Here's how the part is built. I have some questions about the finished solid (model axes, mm). Face numbers are marked on the shaded views. A direction names the side the tool comes from. Round coordinates to 2 decimals unless told otherwise and drop trailing zeros. Loops run counter-clockwise (first coordinate to the right, second up) from the corner with the lowest first, then second, coordinate; pieces in that order, holes last. Notation, with made-up numbers: M 20,47.5 L 44,47.5 A6 cw 44,52.5 Z; hole C 42.25,28.5 d4. An arc over 180 degrees is marked long. Write item = value, one per line. Start each with the question number.
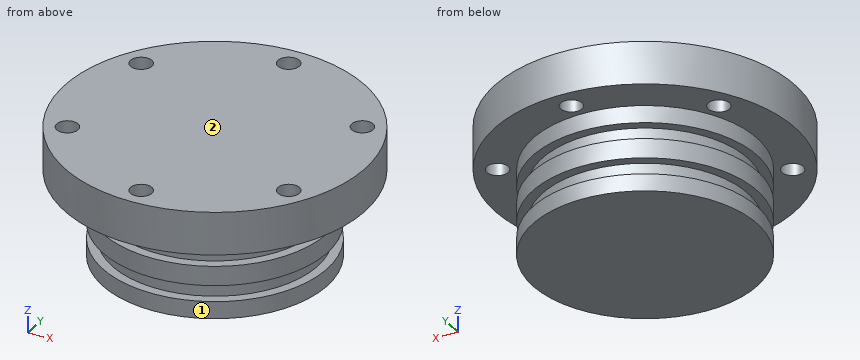
from build123d import *

# Parameters (mm, degrees)
F3_R     = 3.175
F4_DEPTH = 25.4


with BuildPart() as f2:
    # F0 (on Front) → F2 (revolve)
    with BuildSketch(Plane.XZ):
        Polygon((44.45, 38.1), (0, 38.1), (0, 0), (33.2105, 0), (33.2105, 5.08), (30.3911, 5.08), (30.3911, 9.8298), (33.2105, 9.8298), (33.2105, 15.5702), (30.3911, 15.5702), (30.3911, 20.32), (33.2105, 20.32), (33.2105, 25.4), (44.45, 25.4), align=None)
    revolve(axis=Axis((0, 0, 36.677974), (0, 0, -1)))

    # F3 (on face) → F4 (cut)
    with BuildSketch(Plane.XY.offset(38.1)):
        with Locations((0, -38.1)):
            Circle(F3_R)
        with Locations((32.995568, -19.05)):
            Circle(F3_R)
        with Locations((32.995568, 19.05)):
            Circle(F3_R)
        with Locations((0, 38.1)):
            Circle(F3_R)
        with Locations((-32.995568, 19.05)):
            Circle(F3_R)
        with Locations((-32.995568, -19.05)):
            Circle(F3_R)
    extrude(amount=-F4_DEPTH, mode=Mode.SUBTRACT)


solid = f2.part
Item 1: I want a section at C-C, the plane y = 0. List the corners of the cut face in (x, z) for me.
Item 2: I want a section at D-D, the plane x = 32. List the corners of the cut face in (y, z) for me.
Item 3: Will these pins go through, and if not, where does the flat tip stop? pin 1 Ø12 at (y, z) = (2, 13) entering from -X; pin 2 Ø2 at (y, z) = (16, 12) entering from +X; pin 3 Ø4 at (y, z) = (-20.5, 30.5) entering from +X.
Item 4: Please list where these lines run through material, in increasing order: line 1 (Z direction, x = 15.5, y = -28); line 2 (Y direction, x = 0, z = 28.75) (3 decimals); line 3 (X direction, y = -19, z = 30). Write a range as [from, to].
Item 5: I want a section at A-A, the plane x = 0. State how many separate pieces and enclosed holes the cut face has, then the cut area to 3 significant figures.
Item 6: I want a section at B-B, the plane z = 33. List the corners of the cut face in (x, y) for me (3 decimals), then the cut area to 3 significant figures.
Item 7: For the marked faces 1 and 2, which set-ups out of +Z, -Z, +X, -X, +Y, -Y let a thin tool reach every point of the face, with its end or its side?
Worked out:
q1.outline = M -44.45,25.4 L -33.21,25.4 L -33.21,20.32 L -30.39,20.32 L -30.39,15.57 L -33.21,15.57 L -33.21,9.83 L -30.39,9.83 L -30.39,5.08 L -33.21,5.08 L -33.21,0 L 33.21,0 L 33.21,5.08 L 30.39,5.08 L 30.39,9.83 L 33.21,9.83 L 33.21,15.57 L 30.39,15.57 L 30.39,20.32 L 33.21,20.32 L 33.21,25.4 L 44.45,25.4 L 44.45,38.1 L -44.45,38.1 Z
q2.outline = M -30.85,25.4 L -22.06,25.4 L -22.06,38.1 L -30.85,38.1 Z; M -16.04,25.4 L -8.88,25.4 L -8.88,20.32 L 8.88,20.32 L 8.88,25.4 L 16.04,25.4 L 16.04,38.1 L -16.04,38.1 Z; M -8.88,0 L 8.88,0 L 8.88,5.08 L -8.88,5.08 Z; M -8.88,9.83 L 8.88,9.83 L 8.88,15.57 L -8.88,15.57 Z; M 22.06,25.4 L 30.85,25.4 L 30.85,38.1 L 22.06,38.1 Z
q3.pin_1 = -33.21
q3.pin_2 = 29.63
q3.pin_3 = 40.42
q4.line_1 = [0, 5.08], [9.83, 15.57], [20.32, 38.1]
q4.line_2 = [-44.45, -41.275], [-34.925, 34.925], [41.275, 44.45]
q4.line_3 = [-40.18, -36.17], [-29.82, 29.82], [36.17, 40.18]
q5.separate_pieces = 3
q5.enclosed_holes = 0
q5.area = 2,600 mm2
q6.outline = C 0,0 d88.9; hole C -32.996,-19.05 d6.35; hole C -32.996,19.05 d6.35; hole C 0,-38.1 d6.35; hole C 0,38.1 d6.35; hole C 32.996,-19.05 d6.35; hole C 32.996,19.05 d6.35
q6.area = 6,020 mm2
q7.face_1 = -Z
q7.face_2 = +Z, +X, -X, +Y, -Y
